Job drawing, mm, ordinate dimensions from the low corner. One solid piece. A direction names the side the tool comes from. Round coordinates to 2 decimals unless told otherwise and drop trailing zeros. Write each loop counter-clockwise with the first axis right and the second up, starting at its lowest first coordinate (ties: lowest second). Pieces come first, ordered by that corner, then holes.
1) Pull direction Y, two halves, no side cores. Call the marked faces 1, 2, 3 and 4: +Y half, -Y half, draft (parallel to the pull), parting line (faces both ways), or undercut.
2) Flat gauge pins, fed straight in: pin 1 (16 mm diameter, centred on x = 18, y = 43, fed in from -Z); pin 2 (4.5 mm diameter, centred on x = 143, z = 10.5, fed in from -Y); pin 3 (1 mm diameter, centred on y = 34, z = 9.5, fed in from +X); pin 4 (12 mm diameter, centred on y = 15, z = 23, fed in from -X). Where does each tip first touch, or does it go through?
3) Saw through at B-B (x = 176). Write the cut outline in (y, z).
4) Which spindle directions (+Z, -Z, +X, -X, +Y, -Y) get a long thin tool onto all of the face, cutting with end or side? Do the marked faces 5, 6 and 7. Say none if no direction does.
5) Saw through at C-C (z = 31.5). Write the cut outline in (x, y), plus the area to 3 significant figures.
6) Saw through at D-D (y = 27). Write the cut outline in (x, z), plus the area to 3 significant figures.
7) Wall check: probe 1 along Y at (x, z) = (181, 4); probe 2 along X at (y, z) = (39.5, 6); probe 3 along Z at (x, y) = (48, 50). Give the ranges that are in metal, low to high.
8) Saw through at A-A (y = 36). Write the cut outline in (x, z), plus the area to 3 significant figures.
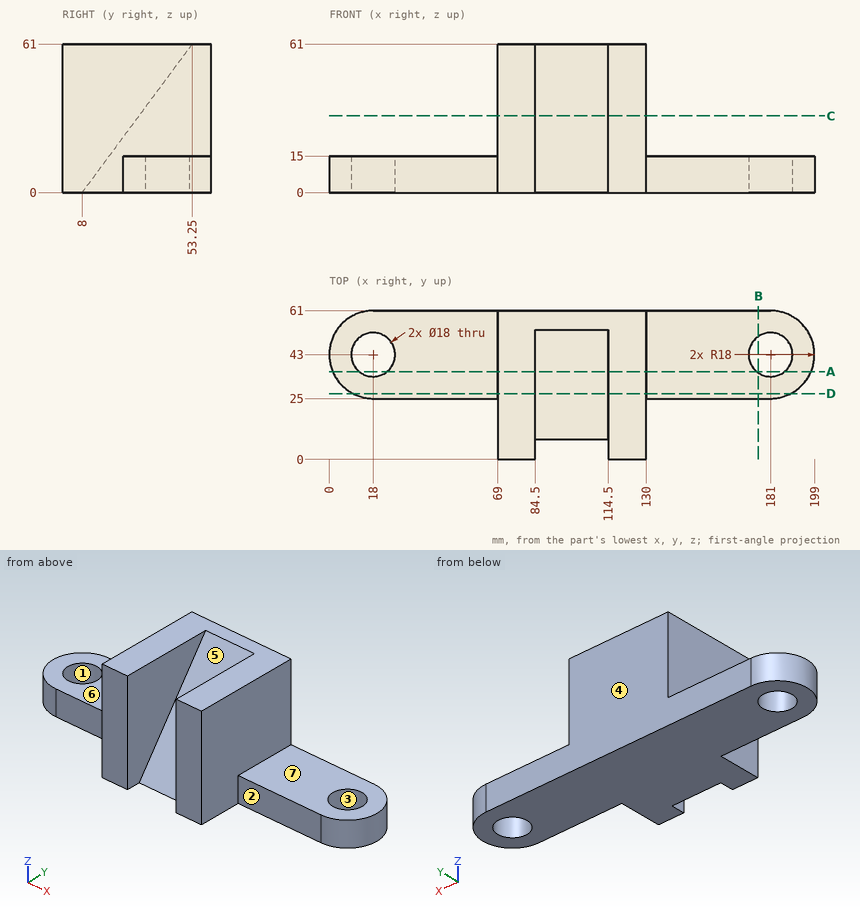
Evaluation:
1. face 1: undercut
1. face 2: -Y half
1. face 3: undercut
1. face 4: +Y half
2. pin 1: passes through
2. pin 2: stops at y = 25
2. pin 3: stops at x = 196.87
2. pin 4: stops at x = 69
3. outline: (25, 0) - (35.52, 0) - (35.52, 15) - (25, 15) - close; (50.48, 0) - (61, 0) - (61, 15) - (50.48, 15) - close
4. face 5: +Z, -Y
4. face 6: +Z, -X, +Y, -Y
4. face 7: +Z, +X, +Y, -Y
5. outline: (69, 0) - (84.5, 0) - (84.5, 31.37) - (114.5, 31.37) - (114.5, 0) - (130, 0) - (130, 61) - (69, 61) - close
5. area: 2,780 mm2
6. outline: (9.75, 0) - (189.25, 0) - (189.25, 15) - (130, 15) - (130, 61) - (114.5, 61) - (114.5, 25.61) - (84.5, 25.61) - (84.5, 61) - (69, 61) - (69, 15) - (9.75, 15) - close
6. area: 4,440 mm2
7. probe 1: y = 25 to 34, 52 to 61
7. probe 2: x = 0.34 to 9.71, 26.29 to 172.71, 189.29 to 198.66
7. probe 3: z = 0 to 15
8. outline: (1.42, 0) - (12.34, 0) - (12.34, 15) - (1.42, 15) - close; (23.66, 0) - (175.34, 0) - (175.34, 15) - (130, 15) - (130, 61) - (114.5, 61) - (114.5, 37.75) - (84.5, 37.75) - (84.5, 61) - (69, 61) - (69, 15) - (23.66, 15) - close; (186.66, 0) - (197.58, 0) - (197.58, 15) - (186.66, 15) - close
8. area: 4,710 mm2
